from build123d import *

# Parameters (mm, degrees)
SKETCH1_R           = 9
BOSS_EXTRUDE1_DEPTH = 50
CUT_EXTRUDE1_DEPTH  = 1
SKETCH3_R           = 9
BOSS_EXTRUDE2_DEPTH = 200


with BuildPart() as part:
    # Sketch1 → Boss-Extrude1 (new, symmetric)
    with BuildSketch(Plane.XY):
        Circle(SKETCH1_R)
    extrude(amount=BOSS_EXTRUDE1_DEPTH, both=True)

    # Sketch2 → Cut-Extrude1 (cut, symmetric)
    with BuildSketch(Plane(origin=(0, 0, 0), x_dir=(0, 0, -1), z_dir=(1, 0, 0))):
        with BuildLine():
            Line((-45, 10.5), (-37, 10.5))
            ThreePointArc((-37, 10.5), (-41, 7.376894374), (-45, 10.5))
        make_face()
    extrude(amount=CUT_EXTRUDE1_DEPTH, both=True, mode=Mode.SUBTRACT)

    # Sketch3 → Boss-Extrude2 (add)
    with BuildSketch(Plane(origin=(0, 0, -50), x_dir=(-1, 0, 0), z_dir=(0, 0, -1))):
        Circle(SKETCH3_R)
    extrude(amount=BOSS_EXTRUDE2_DEPTH)


solid = part.part
Design review of the part built by this model. Coordinates are the model's own, in mm. Coordinates: 2 decimals unless noted, no trailing zeros. Loops run counter-clockwise (first coordinate to the right, second up) from the corner with the lowest first, then second, coordinate; pieces in that order, holes last. Notation, with made-up numbers: M 76,43 L 84,43 A19 ccw 84,65 Z; hole C -13,88.25 d7. An arc over 180 degrees is marked long. Answer as CSV lines item,"result".
Item 1: Add section B-B on x = -4.5. State the section outline as (y, z) points, plus the area to 3 significant figures.
Answer list:
outline,"M -7.79,-250 L 7.79,-250 L 7.79,50 L -7.79,50 Z"
area,"4,680 mm²"
Item 2: For P1, Ø3, axis at x = -2.5, z = -159.5, coming from the +Y side; P2, Ø5, axis at x = 3, z = -185, coming from the -Y side; P3, Ø4, axis at x = 5, z = 2, coming from the -Y side; P4, Ø6, axis at x = 1, z = -160.5, coming from the +Y side, all flat-tipped, find the tip position at first contact; note any pin that passes through.
Answer list:
P1,"y = 8.94"
P2,"y = -8.99"
P3,"y = -8.49"
P4,"y = 9"
Item 3: For probe 1 along Y at (x, z) = (-0.75, -228); probe 2 along X at (y, z) = (7.5, 26.5); probe 3 along Y at (x, z) = (-6.75, -115), list the stretches that pass through material, from the lowest coordinate up.
Answer list:
probe 1,"-8.97 to 8.97"
probe 2,"-4.97 to 4.97"
probe 3,"-5.95 to 5.95"
Item 4: Add section A-A on z = -18. State the section outline as (x, y) points.
Answer list:
outline,"C 0,0 d18"
Item 5: Add section C-C on y = -5.75. State the section outline as (x, z) points.
Answer list:
outline,"M -6.92,-250 L 6.92,-250 L 6.92,50 L -6.92,50 Z"
